For this review, take the finished solid that the model builds, in its own axes (mm). A direction names the side the tool comes from. Round coordinates to 2 decimals unless told otherwise and drop trailing zeros. Order: outer loops, then holes, each group sorted by start corner. A loop starts at its lowest first (then second) coordinate and runs counter-clockwise, first axis right, second up.
from build123d import *

# Parameters (mm, degrees)
IZIM1_R                     = 37.5
IZIM1_R_2                   = 1.75
Y_KSEKLIK_EKSTR_ZYON1_DEPTH = 30


with BuildPart() as part:
    # Çizim1 → Yükseklik-Ekstrüzyon1 (new body)
    with BuildSketch(Plane(origin=(0, 0, 0), x_dir=(1, 0, 0), z_dir=(0, 1, 0))):
        with Locations(Location((0, 0, 0), (0, 0, 270))):
            Circle(IZIM1_R)
        with Locations(Location((0, 35, 0), (0, 0, 270))):
            Circle(IZIM1_R_2, mode=Mode.SUBTRACT)
        with Locations(Location((35, 0, 0), (0, 0, 270))):
            Circle(IZIM1_R_2, mode=Mode.SUBTRACT)
        with Locations(Location((0, -35, 0), (0, 0, 270))):
            Circle(IZIM1_R_2, mode=Mode.SUBTRACT)
        with Locations(Location((-35, 0, 0), (0, 0, 270))):
            Circle(IZIM1_R_2, mode=Mode.SUBTRACT)
        with BuildLine():
            ThreePointArc((-34.771428571, -3.993464048), (-24.748737342, -24.748737342), (-3.993464048, -34.771428571))
            ThreePointArc((-3.993464048, -34.771428571), (0, -31), (3.993464048, -34.771428571))
            ThreePointArc((3.993464048, -34.771428571), (24.748737342, -24.748737342), (34.771428571, -3.993464048))
            ThreePointArc((34.771428571, -3.993464048), (31, 0), (34.771428571, 3.993464048))
            ThreePointArc((34.771428571, 3.993464048), (24.748737342, 24.748737342), (3.993464048, 34.771428571))
            ThreePointArc((3.993464048, 34.771428571), (0, 31), (-3.993464048, 34.771428571))
            ThreePointArc((-3.993464048, 34.771428571), (-24.748737342, 24.748737342), (-34.771428571, 3.993464048))
            ThreePointArc((-34.771428571, 3.993464048), (-31, 0), (-34.771428571, -3.993464048))
        make_face(mode=Mode.SUBTRACT)
    extrude(amount=Y_KSEKLIK_EKSTR_ZYON1_DEPTH)


solid = part.part
(1) Add section D-D on z = -11. Give the boundary of the cut face in (x, y), plus the area to 3 significant figures.
(2) Add section A-A on z = 0. Give the boundary of the cut face in (x, y), plus the area to 3 significant figures.
(3) Add section C-C on x = 21.5. Give the boundary of the cut face in (y, z), plus the area to 3 significant figures.
(4) Add section B-B on y = 12.5. Give the boundary of the cut face in (x, z).
(5) Tool access review of faces 1 (the face through (-33, 0, 0)), 2 (the face through (24.98, 14.79, -24.515)): name each direction out of +Z, -Z, +X, -X, +Y, -Y from which nothing blocks a thin tool from reaching the whole face with its end or side.
(6) Clearance check with flat-ended pins moving along their axes: P1, Ø1.5, axis at x = 11, y = 6.5, coming from the -Z side; P2, Ø1, axis at x = 17, y = 17, coming from the -Z side; P3, Ø3, axis at x = -29, y = 14, coming from the -Z side; P4, Ø2, axis at x = 0, z = 35, coming from the -Y side. State where each tip first meets the part, or that it passes through.
(7) Wall thickness on L1, parallel to Z at x = 13, y = 10.5; L2, parallel to X at y = 10, z = 30.5; L3, parallel to Z at x = -11, y = 19: over which ranges is each line inside the solid? List them lowest first.
Here are the results:
1. outline: (-35.85, 0) - (-33.23, 0) - (-33.23, 30) - (-35.85, 30) - close; (33.23, 0) - (35.85, 0) - (35.85, 30) - (33.23, 30) - close
1. area: 157 mm2
2. outline: (-37.5, 0) - (-36.75, 0) - (-36.75, 30) - (-37.5, 30) - close; (-33.25, 0) - (-31, 0) - (-31, 30) - (-33.25, 30) - close; (31, 0) - (33.25, 0) - (33.25, 30) - (31, 30) - close; (36.75, 0) - (37.5, 0) - (37.5, 30) - (36.75, 30) - close
2. area: 180 mm2
3. outline: (0, -30.72) - (30, -30.72) - (30, -27.62) - (0, -27.62) - close; (0, 27.62) - (30, 27.62) - (30, 30.72) - (0, 30.72) - close
3. area: 186 mm2
4. outline: circle Ø75 at (0, 0); hole circle Ø3.5 at (-35, 0); hole (-34.77, -3.99) arc R35 ccw to (-3.99, -34.77) arc R4 cw to (3.99, -34.77) arc R35 ccw to (34.77, -3.99) arc R4 cw to (34.77, 3.99) arc R35 ccw to (3.99, 34.77) arc R4 cw to (-3.99, 34.77) arc R35 ccw to (-34.77, 3.99) arc R4 cw to start; hole circle Ø3.5 at (0, -35); hole circle Ø3.5 at (0, 35); hole circle Ø3.5 at (35, 0)
5. face 1: +Z, -Z, +X, -X, -Y
5. face 2: +Y, -Y
6. P1: stops at z = -36.07
6. P2: stops at z = -33.67
6. P3: stops at z = -25.5
6. P4: passes through
7. L1: z = -35.17 to -32.5, 32.5 to 35.17
7. L2: x = -21.82 to -17.17, 17.17 to 21.82
7. L3: z = -35.85 to -33.23, 33.23 to 35.85
